from build123d import *

# Parameters (mm, degrees)
F1_DEPTH = 12.5
F2_R     = 1.8
F3_DEPTH = 26
F4_R     = 1.8
F5_DEPTH = 26


with BuildPart() as f1:
    # F0 (on Top) → F1 (new body, symmetric)
    with BuildSketch(Plane.XY):
        with BuildLine():
            ThreePointArc((150, 6), (145.8994949366, 15.8994949366), (136, 20))
            Line((136, 20), (91.7857438326, 20))
            Line((91.7857438326, 20), (116.478802159, -20))
            Line((116.478802159, -20), (136, -20))
            ThreePointArc((136, -20), (145.8994949366, -15.8994949366), (150, -6))
            Line((150, -6), (150, 6))
        make_face()
        with BuildLine():
            Line((26.9902057972, -20), (91.7857438326, 20))
            Line((91.7857438326, 20), (-120.5630078912, 20))
            Line((-120.5630078912, 20), (-136, 20))
            ThreePointArc((-136, 20), (-145.8994949366, 15.8994949366), (-150, 6))
            Line((-150, 6), (-150, -6))
            Line((-150, -6), (-150, -122.7854788303))
            Line((-150, -122.7854788303), (-120.5630078912, -122.7854788303))
            Line((-120.5630078912, -122.7854788303), (-120.5630078912, -20))
            Line((-120.5630078912, -20), (26.9902057972, -20))
        make_face()
        Polygon((116.478802159, -20), (91.7857438326, 20), (26.9902057972, -20), align=None)
        Polygon((116.478802159, -20), (26.9902057972, -20), (-44.4547757506, -64.1048774123), (-20.7777143928, -104.7320792225), align=None)
        Polygon((-20.7777143928, -104.7320792225), (-44.4547757506, -64.1048774123), (-56.7659190817, -71.2796687602), (-33.0888577239, -111.9068705703), align=None)
        Polygon((49.8645024297, -225.9462601459), (-20.7777143928, -104.7320792225), (-33.0888577239, -111.9068705703), (39.7326772195, -236.8605188106), align=None)
        Polygon((-33.0888577239, -111.9068705703), (-56.7659190817, -71.2796687602), (-33.7199519959, -112.2746649823), align=None)
    extrude(amount=F1_DEPTH, both=True)

    # F2 (on face) → F3 (cut)
    with BuildSketch(Plane.XY.offset(12.5)):
        with Locations((-138.6803537607, 0)):
            Circle(F2_R)
    extrude(amount=-F3_DEPTH, mode=Mode.SUBTRACT)

    # F4 (on face) → F5 (cut)
    with BuildSketch(Plane.XY.offset(12.5)):
        with Locations((140.4866278172, 0)):
            Circle(F4_R)
    extrude(amount=-F5_DEPTH, mode=Mode.SUBTRACT)


solid = f1.part
The listing builds one solid part. Answer for the finished solid, in the listing's coordinates (mm). A direction names the side the tool comes from. Coordinates: 2 decimals unless noted, no trailing zeros. Order: outer loops, then holes, each group sorted by start corner. A loop starts at its lowest first (then second) coordinate and runs counter-clockwise, first axis right, second up.
Q1. A cutting plane is placed at A-A, the plane z = 7.75. Write down the section's boundary in (x, y), and give its area (3 significant figures).
Q2. A cutting plane is placed at B-B, the plane x = 12. Write down the section's boundary in (y, z), and give its area (3 significant figures).
Q3. Consider line 1 (Y direction, x = 5, z = 4); line 2 (Y direction, x = 11, z = 7.5); line 3 (Y direction, x = -134, z = -7). Determine where each line is inside the solid, lowest interval first.
Q4. A cutting plane is placed at D-D, the plane y = -139. Write down the section's boundary in (x, z).
Q5. Which of the six approach directions +Z, -Z, +X, -X, +Y, -Y give full straight-line access (tool end or side, diameter ignored) to faces 1 (the face through (-135, -122.785, 0)), 2 (the face through (-48, -20, 0)), 3 (the face through (15.04, -166.19, 0.18)), 4 (the face through (-120.563, -72, 0)), 5 (the face through (126, -20, 0))?
Q6. For a pull along X with two mould halves and no side action, classify faces 6 (the face through (-12, -60, -12.5)), 7 (the face through (146, 15.8, 0.2)), 8 (the face through (-8.232, -41.744, 0.175)) as pulls with the +X half, pulls with the -X half, needs draft (parallel to the pull), parting line crosses it, or undercut.
Q7. A cutting plane is placed at C-C, the plane y = -29. Write down the section's boundary in (x, z), and give its area (3 significant figures).
Q8. Given P1, Ø5, axis at y = -99.5, z = 8.5, coming from the +X side; P2, Ø10, axis at x = 126.5, z = 4, coming from the -Y side; P3, Ø3, axis at x = 140.49, y = 0, coming from the -Z side; P4, Ø7.5, axis at x = -21, z = 6, coming from the -Y side, each flat-ended and moving along its own axis, determine where each tip first touches the part or whether it passes through.
Answers follow:
1. outline: (-150, -122.79) - (-120.56, -122.79) - (-120.56, -20) - (26.99, -20) - (-44.45, -64.1) - (-56.77, -71.28) - (-33.72, -112.27) - (-33.09, -111.91) - (39.73, -236.86) - (49.86, -225.95) - (-20.78, -104.73) - (116.48, -20) - (136, -20) arc R14 ccw to (150, -6) - (150, 6) arc R14 ccw to (136, 20) - (-136, 20) arc R14 ccw to (-150, 6) - close; hole circle Ø3.6 at (-138.68, 0); hole circle Ø3.6 at (140.49, 0)
1. area: 23,400 mm2
2. outline: (-189.27, -12.5) - (-160.97, -12.5) - (-160.97, 12.5) - (-189.27, 12.5) - close; (-84.5, -12.5) - (-29.25, -12.5) - (-29.25, 12.5) - (-84.5, 12.5) - close; (-20, -12.5) - (20, -12.5) - (20, 12.5) - (-20, 12.5) - close
2. area: 3,090 mm2
3. line 1: y = -177.26 to -148.96, -88.82 to -33.58, -20 to 20
3. line 2: y = -187.56 to -159.26, -85.11 to -29.87, -20 to 20
3. line 3: y = -122.79 to 20
4. outline: (-17.3, -12.5) - (-0.81, -12.5) - (-0.81, 12.5) - (-17.3, 12.5) - close
5. face 1: +Z, -Z, -X, -Y
5. face 2: +Z, -Z
5. face 3: +Z, -Z, +X
5. face 4: +Z, -Z, -Y
5. face 5: +Z, -Z, +X, -Y
6. face 6: needs draft
6. face 7: pulls with the +X half
6. face 8: undercut
7. outline: (-150, -12.5) - (-120.56, -12.5) - (-120.56, 12.5) - (-150, 12.5) - close; (12.41, -12.5) - (101.9, -12.5) - (101.9, 12.5) - (12.41, 12.5) - close
7. area: 2,970 mm2
8. P1: stops at x = -8.25
8. P2: stops at y = -20
8. P3: passes through
8. P4: stops at y = -139.08
